Design review of the part built by this model. Coordinates are the model's own, in mm. A direction names the side the tool comes from. Coordinates: 2 decimals unless noted, no trailing zeros. Loops run counter-clockwise (first coordinate to the right, second up) from the corner with the lowest first, then second, coordinate; pieces in that order, holes last. Notation, with made-up numbers: (62.5, 28.5) - (78.5, 28.5) arc R27 ccw to (78.5, 53.5) - close; hole circle Ø8 at (11, 47.25). An arc over 180 degrees is marked (long way). Answer in a Markdown table with one row per item. Add a question column.
(1) For faces 1 (the face through (95, -5, 15)), 2 (the face through (-96, 0, 9)), 3 (the face through (-64, 0, 1)), 4 (the face through (-86.015, -24.58, 13.339)), list the 3-axis set-ups (+Z, -Z, +X, -X, +Y, -Y) from which the entire face can be reached by the end or side of a thin tool; tool diameter is ignored.
(2) We need section B-B, the plane x = 16. Write out the cut boundary in (y, z).
(3) To check wall thickness, follow L1, parallel to Y at x = -67.5, z = 3.75; L2, parallel to X at y = 6.5, z = 19.75; L3, parallel to Y at x = -16, z = 0.75. State the ranges of each line that lie inside material, in increasing order. Write a range as [from, to].
(4) We need section C-C, the plane y = -25. Give the number of separate pieces and of enclosed holes in the cut face, plus the area to 3 significant figures.
(5) The part is to be moulded in two halves that separate along Y. For faces 5 (the face through (54.445, -12.03, 0.986)), 6 (the face through (-96, 0, 22)), say which applies: released by +Y, released by -Y, zero draft, split by the parting line, or undercut.
(6) We need section A-A, the plane z = 10. Write out the cut boundary in (x, y), plus the area to 3 significant figures.
(7) Clearance check with flat-ended pins moving along their axes: pin 1 (1.5 mm diameter, centred on x = 53.5, y = -7.5, fed in from +Z); pin 2 (1.5 mm diameter, centred on x = -49, z = 14, fed in from +Y); pin 3 (2.5 mm diameter, centred on y = 0, z = 23, fed in from +X); pin 4 (4 mm diameter, centred on x = 16, y = -25, fed in from -Z). State where each tip first meets the part, or that it passes through.
from build123d import *

# Parameters (mm, degrees)
F1_DEPTH  = 25
F2_T      = -2
F3_W      = 1
F3_H      = 20
F4_DEPTH  = 192.001
F5_W      = 10
F5_H      = 5
F6_DEPTH  = 2
F8_DEPTH  = 40.001
F9_W      = 10
F9_H      = 5
F10_DEPTH = 2
F12_DEPTH = 40.001
F13_W     = 2
F13_H     = 12.5
F14_DEPTH = 1
F16_DEPTH = 159.001
F17_W     = 2
F17_H     = 12.5
F18_DEPTH = 1
F20_DEPTH = 159.001
F21_R     = 2.6
F22_DEPTH = 25.001
F23_W     = 11
F23_H     = 29
F24_DEPTH = 25.001
F25_R     = 3


with BuildPart() as f1:
    # F0 (on Top) → F1 (new body)
    with BuildSketch(Plane.XY):
        with BuildLine():
            ThreePointArc((-66, 35), (-87.213203, 26.213203), (-96, 5))
            Line((-96, 5), (-96, -5))
            ThreePointArc((-96, -5), (-87.213203, -26.213203), (-66, -35))
            Line((-66, -35), (66, -35))
            ThreePointArc((66, -35), (87.213203, -26.213203), (96, -5))
            Line((96, -5), (96, 5))
            ThreePointArc((96, 5), (87.213203, 26.213203), (66, 35))
            Line((66, 35), (-66, 35))
        make_face()
    extrude(amount=F1_DEPTH)

    # F2
    f2_openings = [f1.faces().sort_by_distance(p)[0] for p in [
        (0, 0, 25),
    ]]
    offset(amount=F2_T, openings=f2_openings)

    # F3 (on face) → F4 (cut, through all)
    with BuildSketch(Plane.YZ.offset(96)):
        with Locations((-5.5, 15)):
            Rectangle(F3_W, F3_H)
        with Locations((5.5, 15)):
            Rectangle(F3_W, F3_H)
    extrude(amount=-F4_DEPTH, mode=Mode.SUBTRACT)

    # F5 (on face) → F6 (join)
    with BuildSketch(Plane.YZ.offset(96)):
        with Locations((0, 17.5)):
            Rectangle(F5_W, F5_H)
    extrude(amount=F6_DEPTH)

    # F7 (on face) → F8 (cut, through all)
    with BuildSketch(Plane.XZ.offset(5)):
        Polygon((97, 20), (98, 15), (98, 20), align=None)
    extrude(amount=-F8_DEPTH, mode=Mode.SUBTRACT)

    # F9 (on face) → F10 (join)
    with BuildSketch(Plane(origin=(-96, 0, 0), x_dir=(0, -1, 0), z_dir=(-1, 0, 0))):
        with Locations((0, 17.5)):
            Rectangle(F9_W, F9_H)
    extrude(amount=F10_DEPTH)

    # F11 (on face) → F12 (cut, through all)
    with BuildSketch(Plane(origin=(0, 5, 0), x_dir=(-1, 0, 0), z_dir=(0, 1, 0))):
        Polygon((97, 20), (98, 15), (98, 20), align=None)
    extrude(amount=-F12_DEPTH, mode=Mode.SUBTRACT)

    # F13 (on face) → F14 (join)
    with BuildSketch(Plane.XZ.offset(35)):
        with Locations((-60, 18.75)):
            Rectangle(F13_W, F13_H)
        with Locations((0, 18.75)):
            Rectangle(F13_W, F13_H)
        with Locations((60, 18.75)):
            Rectangle(F13_W, F13_H)
    extrude(amount=F14_DEPTH)

    # F15 (on face) → F16 (cut, through all)
    with BuildSketch(Plane.YZ.offset(61)):
        Polygon((-36, 12.5), (-35, 12.5), (-36, 18.75), align=None)
    extrude(amount=-F16_DEPTH, mode=Mode.SUBTRACT)

    # F17 (on face) → F18 (join)
    with BuildSketch(Plane(origin=(0, 35, 0), x_dir=(-1, 0, 0), z_dir=(0, 1, 0))):
        with Locations((-60, 18.75)):
            Rectangle(F17_W, F17_H)
        with Locations((0, 18.75)):
            Rectangle(F17_W, F17_H)
        with Locations((60, 18.75)):
            Rectangle(F17_W, F17_H)
    extrude(amount=F18_DEPTH)

    # F19 (on face) → F20 (cut, through all)
    with BuildSketch(Plane(origin=(-61, 0, 0), x_dir=(0, -1, 0), z_dir=(-1, 0, 0))):
        Polygon((-36, 12.5), (-35, 12.5), (-36, 18.75), align=None)
    extrude(amount=-F20_DEPTH, mode=Mode.SUBTRACT)

    # F21 (on face) → F22 (cut, through all)
    with BuildSketch(Plane(origin=(0, 0, 0), x_dir=(1, 0, 0), z_dir=(0, 0, -1))):
        with Locations((-66, 25)):
            Circle(F21_R)
        with Locations((-16, 25)):
            Circle(F21_R)
        with Locations((-66, -25)):
            Circle(F21_R)
        with Locations((-16, -25)):
            Circle(F21_R)
        with BuildLine():
            Line((-31.124102, 11.290112), (-26.87471, 15.539504))
            ThreePointArc((-26.87471, 15.539504), (-41, 21), (-55.12529, 15.539504))
            Line((-55.12529, 15.539504), (-50.875898, 11.290112))
            ThreePointArc((-50.875898, 11.290112), (-41, 15), (-31.124102, 11.290112))
        make_face()
        with BuildLine():
            ThreePointArc((-25.460496, -14.12529), (-20, 0), (-25.460496, 14.12529))
            Line((-25.460496, 14.12529), (-29.709888, 9.875898))
            ThreePointArc((-29.709888, 9.875898), (-26, 0), (-29.709888, -9.875898))
            Line((-29.709888, -9.875898), (-25.460496, -14.12529))
        make_face()
        with BuildLine():
            ThreePointArc((-55.12529, -15.539504), (-41, -21), (-26.87471, -15.539504))
            Line((-26.87471, -15.539504), (-31.124102, -11.290112))
            ThreePointArc((-31.124102, -11.290112), (-41, -15), (-50.875898, -11.290112))
            Line((-50.875898, -11.290112), (-55.12529, -15.539504))
        make_face()
        with BuildLine():
            ThreePointArc((-56.539504, 14.12529), (-62, 0), (-56.539504, -14.12529))
            Line((-56.539504, -14.12529), (-52.290112, -9.875898))
            ThreePointArc((-52.290112, -9.875898), (-56, 0), (-52.290112, 9.875898))
            Line((-52.290112, 9.875898), (-56.539504, 14.12529))
        make_face()
        with BuildLine():
            Line((-60.786795, 21.201008), (-56.54097, 16.955184))
            ThreePointArc((-56.54097, 16.955184), (-41, 23), (-25.45903, 16.955184))
            Line((-25.45903, 16.955184), (-21.213205, 21.201008))
            ThreePointArc((-21.213205, 21.201008), (-41, 29), (-60.786795, 21.201008))
        make_face()
        with BuildLine():
            Line((-21.213205, -21.201008), (-25.45903, -16.955184))
            ThreePointArc((-25.45903, -16.955184), (-41, -23), (-56.54097, -16.955184))
            Line((-56.54097, -16.955184), (-60.786795, -21.201008))
            ThreePointArc((-60.786795, -21.201008), (-41, -29), (-21.213205, -21.201008))
        make_face()
        with BuildLine():
            Line((-62.201008, -19.786795), (-57.955184, -15.54097))
            ThreePointArc((-57.955184, -15.54097), (-64, 0), (-57.955184, 15.54097))
            Line((-57.955184, 15.54097), (-62.201008, 19.786795))
            ThreePointArc((-62.201008, 19.786795), (-70, 0), (-62.201008, -19.786795))
        make_face()
        with BuildLine():
            Line((-19.798992, 19.786795), (-24.044816, 15.54097))
            ThreePointArc((-24.044816, 15.54097), (-18, 0), (-24.044816, -15.54097))
            Line((-24.044816, -15.54097), (-19.798992, -19.786795))
            ThreePointArc((-19.798992, -19.786795), (-12, 0), (-19.798992, 19.786795))
        make_face()
        with Locations((16, 25)):
            Circle(F21_R)
        with Locations((66, 25)):
            Circle(F21_R)
        with Locations((16, -25)):
            Circle(F21_R)
        with Locations((66, -25)):
            Circle(F21_R)
        with BuildLine():
            Line((50.875898, 11.290112), (55.12529, 15.539504))
            ThreePointArc((55.12529, 15.539504), (41, 21), (26.87471, 15.539504))
            Line((26.87471, 15.539504), (31.124102, 11.290112))
            ThreePointArc((31.124102, 11.290112), (41, 15), (50.875898, 11.290112))
        make_face()
        with BuildLine():
            ThreePointArc((56.539504, -14.12529), (62, 0), (56.539504, 14.12529))
            Line((56.539504, 14.12529), (52.290112, 9.875898))
            ThreePointArc((52.290112, 9.875898), (56, 0), (52.290112, -9.875898))
            Line((52.290112, -9.875898), (56.539504, -14.12529))
        make_face()
        with BuildLine():
            ThreePointArc((26.87471, -15.539504), (41, -21), (55.12529, -15.539504))
            Line((55.12529, -15.539504), (50.875898, -11.290112))
            ThreePointArc((50.875898, -11.290112), (41, -15), (31.124102, -11.290112))
            Line((31.124102, -11.290112), (26.87471, -15.539504))
        make_face()
        with BuildLine():
            ThreePointArc((25.460496, 14.12529), (20, 0), (25.460496, -14.12529))
            Line((25.460496, -14.12529), (29.709888, -9.875898))
            ThreePointArc((29.709888, -9.875898), (26, 0), (29.709888, 9.875898))
            Line((29.709888, 9.875898), (25.460496, 14.12529))
        make_face()
        with BuildLine():
            Line((21.213205, 21.201008), (25.45903, 16.955184))
            ThreePointArc((25.45903, 16.955184), (41, 23), (56.54097, 16.955184))
            Line((56.54097, 16.955184), (60.786795, 21.201008))
            ThreePointArc((60.786795, 21.201008), (41, 29), (21.213205, 21.201008))
        make_face()
        with BuildLine():
            Line((60.786795, -21.201008), (56.54097, -16.955184))
            ThreePointArc((56.54097, -16.955184), (41, -23), (25.45903, -16.955184))
            Line((25.45903, -16.955184), (21.213205, -21.201008))
            ThreePointArc((21.213205, -21.201008), (41, -29), (60.786795, -21.201008))
        make_face()
        with BuildLine():
            Line((19.798992, -19.786795), (24.044816, -15.54097))
            ThreePointArc((24.044816, -15.54097), (18, 0), (24.044816, 15.54097))
            Line((24.044816, 15.54097), (19.798992, 19.786795))
            ThreePointArc((19.798992, 19.786795), (12, 0), (19.798992, -19.786795))
        make_face()
        with BuildLine():
            Line((62.201008, 19.786795), (57.955184, 15.54097))
            ThreePointArc((57.955184, 15.54097), (64, 0), (57.955184, -15.54097))
            Line((57.955184, -15.54097), (62.201008, -19.786795))
            ThreePointArc((62.201008, -19.786795), (70, 0), (62.201008, 19.786795))
        make_face()
    extrude(amount=-F22_DEPTH, mode=Mode.SUBTRACT)

    # F23 (on face) → F24 (cut, through all)
    with BuildSketch(Plane(origin=(0, 0, 0), x_dir=(1, 0, 0), z_dir=(0, 0, -1))):
        Rectangle(F23_W, F23_H)
    extrude(amount=-F24_DEPTH, mode=Mode.SUBTRACT)

    # F25
    f25_edges = [f1.edges().sort_by_distance(p)[0] for p in [
        (87.213203, 26.213203, 0),
    ]]
    fillet(f25_edges, radius=F25_R)


solid = f1.part
Responses:
| question | item | result |
|---|---|---|
| 1 | face 1 | +Z, +X, -X |
| 1 | face 2 | -Z, -X, +Y, -Y |
| 1 | face 3 | +Z, -Z |
| 1 | face 4 | +Z |
| 2 | outline | (-35, 3) arc R3 ccw to (-32, 0) - (-27.6, 0) - (-27.6, 2) - (-33, 2) - (-33, 25) - (-35, 25) - close; (-22.4, 0) - (-14.7, 0) - (-14.7, 2) - (-22.4, 2) - close; (14.7, 0) - (22.4, 0) - (22.4, 2) - (14.7, 2) - close; (27.6, 0) - (32, 0) arc R3 ccw to (35, 3) - (35, 25) - (33, 25) - (33, 2) - (27.6, 2) - close |
| 3 | L1 | y = [-34.96, -32.96], [32.96, 34.96] |
| 3 | L2 | x = [-95.96, -93.96], [93.96, 95.96] |
| 3 | L3 | y = [-33.98, -27.6], [-22.4, -14.7], [14.7, 22.4], [27.6, 33.98] |
| 4 | separate pieces | 7 |
| 4 | enclosed holes | 0 |
| 4 | area | 316 mm2 |
| 5 | face 5 | undercut |
| 5 | face 6 | zero draft |
| 6 | outline | (-96, -5) - (-94, -5) - (-94, 5) - (-96, 5) - close; (-95.98, -6) arc R30 ccw to (-66, -35) - (66, -35) arc R30 ccw to (95.98, -6) - (93.98, -6) arc R28 cw to (66, -33) - (-66, -33) arc R28 cw to (-93.98, -6) - close; (-95.98, 6) - (-93.98, 6) arc R28 cw to (-66, 33) - (66, 33) arc R28 cw to (93.98, 6) - (95.98, 6) arc R30 ccw to (66, 35) - (-66, 35) arc R30 ccw to start; (94, -5) - (96, -5) - (96, 5) - (94, 5) - close |
| 6 | area | 924 mm2 |
| 7 | pin 1 | stops at z = 2 |
| 7 | pin 2 | stops at y = 35 |
| 7 | pin 3 | stops at x = 96 |
| 7 | pin 4 | passes through |
